Source: CAD feature listing. Evaluate the final solid. Frame: model axes, mm. Face numbers are marked on the shaded views. Coordinates: 2 decimals unless noted, no trailing zeros. Loops run counter-clockwise (first coordinate to the right, second up) from the corner with the lowest first, then second, coordinate; pieces in that order, holes last. Notation, with made-up numbers: (-8.75, 46) - (25.25, 46) arc R22 cw to (25.25, 65) - close; hole circle Ø10 at (9, 83). An arc over 180 degrees is marked (long way). Write item = value, one per line. Start each with the question number.
from build123d import *

# Parameters (mm, degrees)
F0_W     = 50
F0_H     = 50
F1_DEPTH = 80
F2_R     = 10
F3_DEPTH = 50


with BuildPart() as f1:
    # F0 (on Right) → F1 (new body)
    with BuildSketch(Plane.YZ):
        Rectangle(F0_W, F0_H)
    extrude(amount=-F1_DEPTH)

    # F2 (on face) → F3 (cut, through all)
    with BuildSketch(Plane.XZ.offset(25)):
        with Locations((-60, 10)):
            Circle(F2_R)
        with Locations((-20, 10)):
            Circle(F2_R)
    extrude(amount=-F3_DEPTH, mode=Mode.SUBTRACT)


solid = f1.part
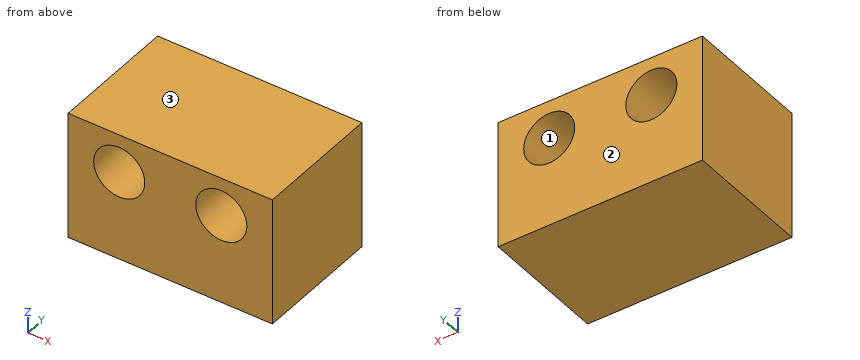
Item 1: Cut plane C-C (y = -19). Return the cut outline in (x, z), then the cut area to 3 significant figures.
Item 2: Draft query along Z for the marked faces 1, 2 and 3. Return one class per face: released by +Z, released by -Z, zero draft, split by the parting line, or undercut.
Item 3: Cut plane D-D (x = -28). Return the cut outline in (y, z), then the cut area to 3 significant figures.
Item 4: Cut plane A-A (z = 10). Return the cut outline in (x, y), then the cut area to 3 significant figures.
Item 5: Material intervals for L1, parallel to Z at x = -59.5, y = -2; L2, parallel to X at y = -9, z = 11; L3, parallel to Z at x = -66, y = 10, sorted ascending. Write a range as [from, to].
Item 6: Cut plane B-B (x = -60). Return the cut outline in (y, z).
Responses:
q1.outline = (-80, -25) - (0, -25) - (0, 25) - (-80, 25) - close; hole circle Ø20 at (-60, 10); hole circle Ø20 at (-20, 10)
q1.area = 3,370 mm2
q2.face_1 = undercut
q2.face_2 = zero draft
q2.face_3 = released by +Z
q3.outline = (-25, -25) - (25, -25) - (25, 4) - (-25, 4) - close; (-25, 16) - (25, 16) - (25, 25) - (-25, 25) - close
q3.area = 1,900 mm2
q4.outline = (-80, -25) - (-70, -25) - (-70, 25) - (-80, 25) - close; (-50, -25) - (-30, -25) - (-30, 25) - (-50, 25) - close; (-10, -25) - (0, -25) - (0, 25) - (-10, 25) - close
q4.area = 2,000 mm2
q5.L1 = [-25, 0.01], [19.99, 25]
q5.L2 = [-80, -69.95], [-50.05, -29.95], [-10.05, 0]
q5.L3 = [-25, 2], [18, 25]
q6.outline = (-25, -25) - (25, -25) - (25, 0) - (-25, 0) - close; (-25, 20) - (25, 20) - (25, 25) - (-25, 25) - close
